Design review of the part shown in the three views and the two pictorial views. Dimensions are in mm from the part's minimum x, y and z. Coordinates: 2 decimals unless noted, no trailing zeros. Loops run counter-clockwise (first coordinate to the right, second up) from the corner with the lowest first, then second, coordinate; pieces in that order, holes last. Notation, with made-up numbers: M 59,61.25 L 110,61.25 A26 cw 110,83.25 Z; hole C -8,53 d4. An arc over 180 degrees is marked long. Use one line per item in the form item = value.
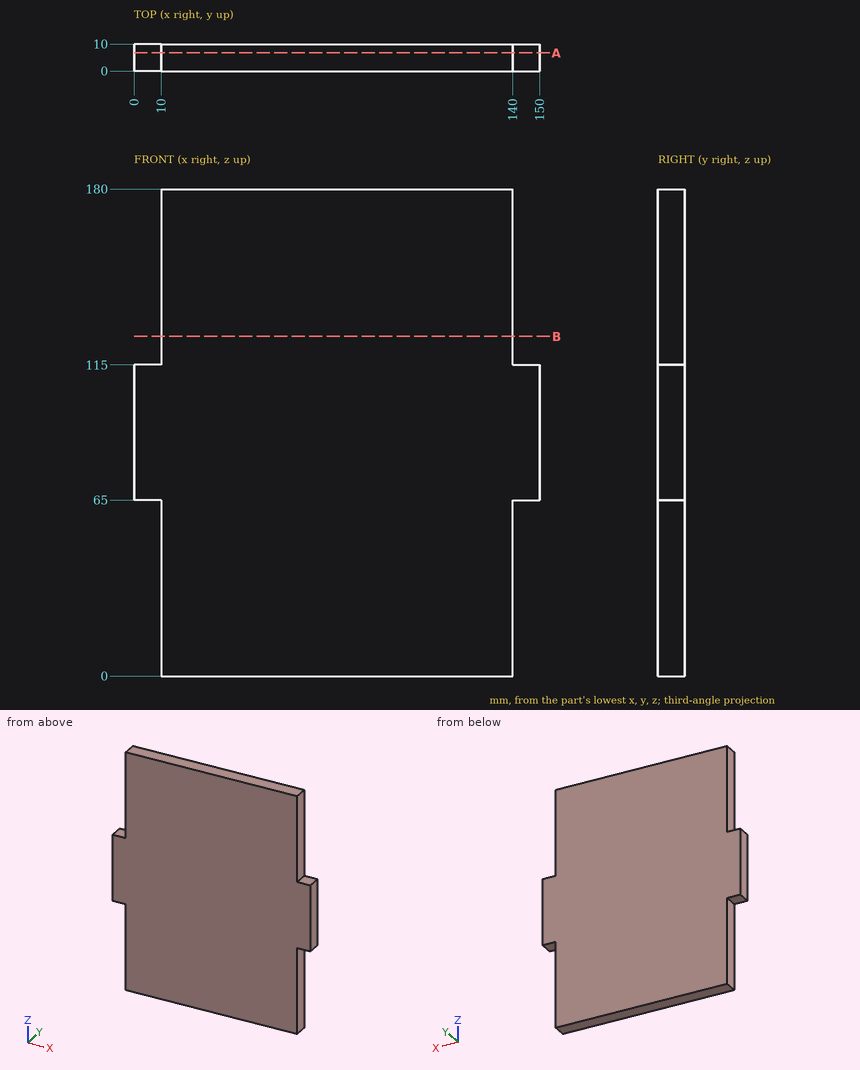
1. Add section B-B (z = 125.5). State the section outline as (x, y) points, then the cut area to 3 significant figures.
Response values:
outline = M 10,0 L 140,0 L 140,10 L 10,10 Z
area = 1,300 mm^2
2. Wall thickness on line 1 along X through (y, z) = (4, 46); line 2 along Z through (x, y) = (141, 8): over which ranges is each line inside the solid? List them lowest first. Write a range as from..to.
Response values:
line_1 = 10..140
line_2 = 65..115
3. Add section A-A (y = 6.75). State the section outline as (x, z) points.
Response values:
outline = M 0,65 L 10,65 L 10,0 L 140,0 L 140,65 L 150,65 L 150,115 L 140,115 L 140,180 L 10,180 L 10,115 L 0,115 Z
4. Insertion check: P1, Ø3, axis at y = 4, z = 134.5, coming from the +X side; P2, Ø2, axis at x = 18.5, z = 148, coming from the -Y side; P3, Ø3, axis at x = 4, y = 6.5, coming from the +Z side; P4, Ø5, axis at y = 7, z = 145, coming from the -X side. Each pin has a flat end and moves straight along its axis. Give the tip position at first contact, or say it passes through.
Response values:
P1 = 140
P2 = 0
P3 = 115
P4 = 10
